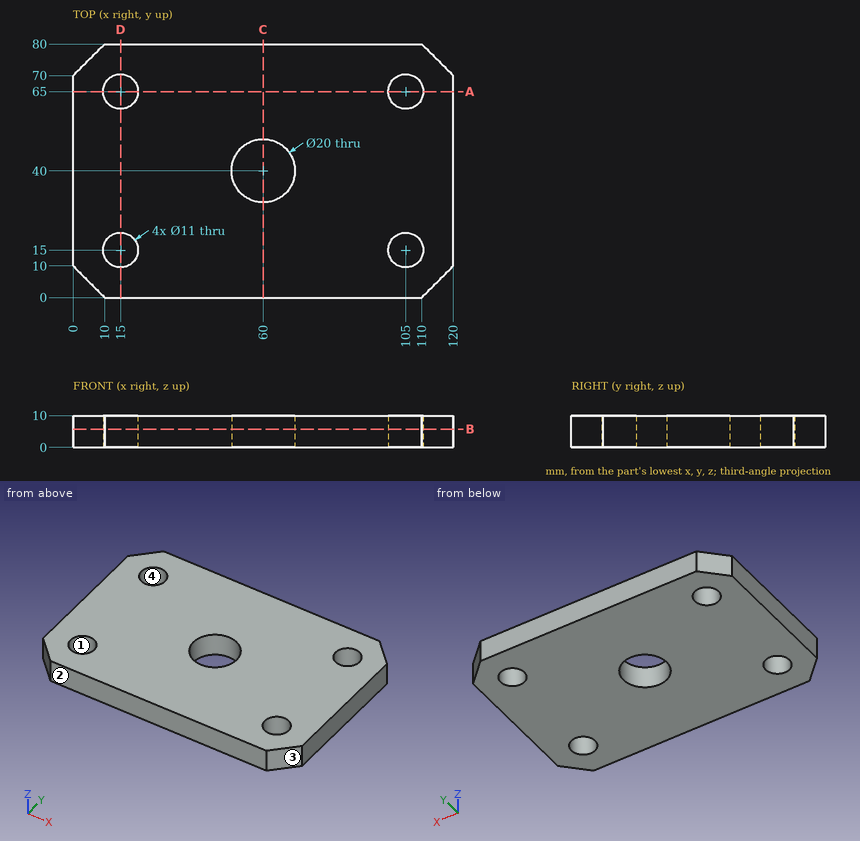
Geometry check sheet. Reference: drawing and pictorial views, mm from the part's lowest x, y, z. Coordinates: 2 decimals unless noted, no trailing zeros. Order: outer loops, then holes, each group sorted by start corner. A loop starts at its lowest first (then second) coordinate and runs counter-clockwise, first axis right, second up. Notation, with made-up numbers: (44, -7.5) - (91, -7.5) arc R14 ccw to (91, 10.5) - close; hole circle Ø10 at (35, 38.5). An arc over 180 degrees is marked (long way). Answer in a Markdown table with one row per item. Add a question column.
1) Release check for a two-part mould opening along X. For the marked faces 1, 2, 3 and 4 record: +X half, -X half, draft (parallel to the pull), parting line (faces both ways), or undercut.
2) Gauge pin test, flat ends, axial feed: P1, Ø14.5, axis at x = 15, y = 65, coming from the -Z side; P2, Ø2, axis at y = 8, z = 4.5, coming from the -X side. Record the tip position at first contact, or that the pin passes through.
3) Cross-section at B-B, the plane z = 5.75. Record the cut outline in (x, y).
4) Cross-section at C-C, the plane x = 60. Record the cut outline in (y, z), then the cut area to 3 significant figures.
5) Material ranges on line 1 along Y through (x, z) = (105, 6); line 2 along X through (y, z) = (70, 2.25); line 3 along Y through (x, z) = (60, 4.5), recorded low to high. Write a range as [from, to].
6) Cross-section at D-D, the plane x = 15. Record the cut outline in (y, z), then the cut area to 3 significant figures.
7) Cross-section at A-A, the plane y = 65. Record the cut outline in (x, z), then the cut area to 3 significant figures.
Check result:
| question | item | result |
|---|---|---|
| 1 | face 1 | undercut |
| 1 | face 2 | draft |
| 1 | face 3 | +X half |
| 1 | face 4 | undercut |
| 2 | P1 | stops at z = 0 |
| 2 | P2 | stops at x = 1 |
| 3 | outline | (0, 10) - (10, 0) - (110, 0) - (120, 10) - (120, 70) - (110, 80) - (10, 80) - (0, 70) - close; hole circle Ø11 at (15, 15); hole circle Ø11 at (15, 65); hole circle Ø20 at (60, 40); hole circle Ø11 at (105, 15); hole circle Ø11 at (105, 65) |
| 4 | outline | (0, 0) - (30, 0) - (30, 10) - (0, 10) - close; (50, 0) - (80, 0) - (80, 10) - (50, 10) - close |
| 4 | area | 600 mm² |
| 5 | line 1 | y = [0, 9.5], [20.5, 59.5], [70.5, 80] |
| 5 | line 2 | x = [0, 12.71], [17.29, 102.71], [107.29, 120] |
| 5 | line 3 | y = [0, 30], [50, 80] |
| 6 | outline | (0, 0) - (9.5, 0) - (9.5, 10) - (0, 10) - close; (20.5, 0) - (59.5, 0) - (59.5, 10) - (20.5, 10) - close; (70.5, 0) - (80, 0) - (80, 10) - (70.5, 10) - close |
| 6 | area | 580 mm² |
| 7 | outline | (0, 0) - (9.5, 0) - (9.5, 10) - (0, 10) - close; (20.5, 0) - (99.5, 0) - (99.5, 10) - (20.5, 10) - close; (110.5, 0) - (120, 0) - (120, 10) - (110.5, 10) - close |
| 7 | area | 980 mm² |
